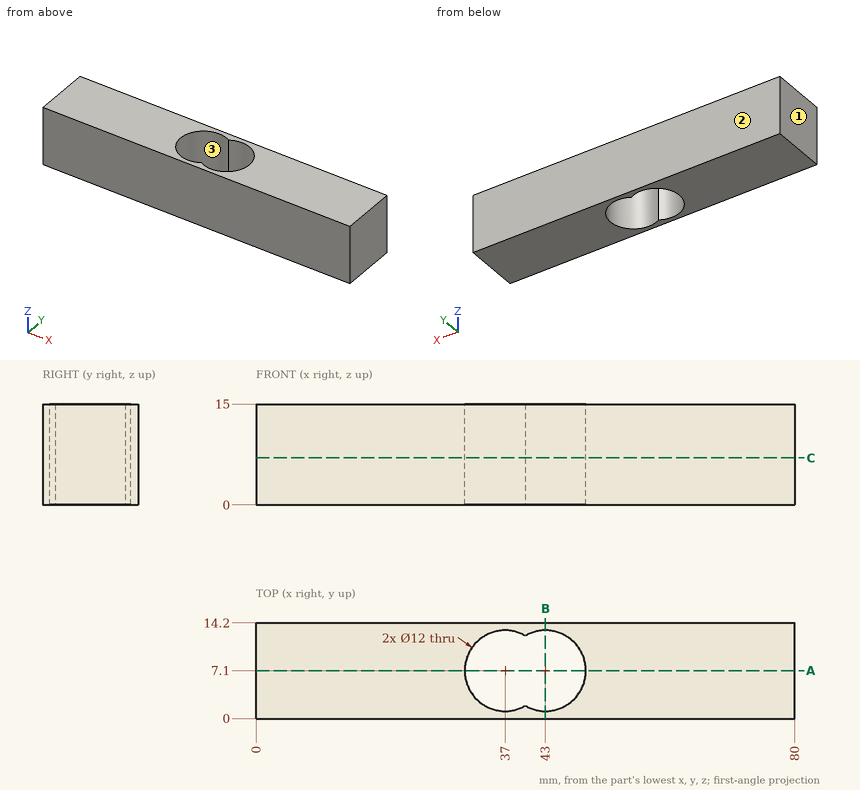
Could you check a few things on this drawing? It's one solid part, dimensions in mm from its lowest x, y, z. Round coordinates to 2 decimals unless told otherwise and drop trailing zeros. Write each loop counter-clockwise with the first axis right and the second up, starting at its lowest first coordinate (ties: lowest second). Pieces come first, ordered by that corner, then holes.
Q1. If we section it at B-B on x = 43: Write out the boundary of the cut face in (y, z), plus the area to 3 significant figures.
Q2. If we section it at C-C on z = 7: Write out the boundary of the cut face in (x, y), plus the area to 3 significant figures.
Q3. If we section it at A-A on y = 7.1: Write out the boundary of the cut face in (x, z).
Q4. If we mould it in two halves opening along X, with no side actions, what happens to the marked faces 1, 2 and 3? For each: +X half, -X half, draft (parallel to the pull), parting line (faces both ways), or undercut.
Q5. Please list where these lines run through material, in increasing order: probe 1 along Y at (x, z) = (37, 3.75); probe 2 along X at (y, z) = (7.5, 12.25); probe 3 along X at (y, z) = (8.5, 6.5).
Answer below:
1. outline: (0, 0) - (1.1, 0) - (1.1, 15) - (0, 15) - close; (13.1, 0) - (14.2, 0) - (14.2, 15) - (13.1, 15) - close
1. area: 33.0 mm2
2. outline: (0, 0) - (80, 0) - (80, 14.2) - (0, 14.2) - close; hole (40, 1.9) arc R6 ccw (long way) to (40, 12.3) arc R6 ccw (long way) to start
2. area: 954 mm2
3. outline: (0, 0) - (31, 0) - (31, 15) - (0, 15) - close; (49, 0) - (80, 0) - (80, 15) - (49, 15) - close
4. face 1: -X half
4. face 2: draft
4. face 3: undercut
5. probe 1: y = 0 to 1.1, 13.1 to 14.2
5. probe 2: x = 0 to 31.01, 48.99 to 80
5. probe 3: x = 0 to 31.17, 48.83 to 80
